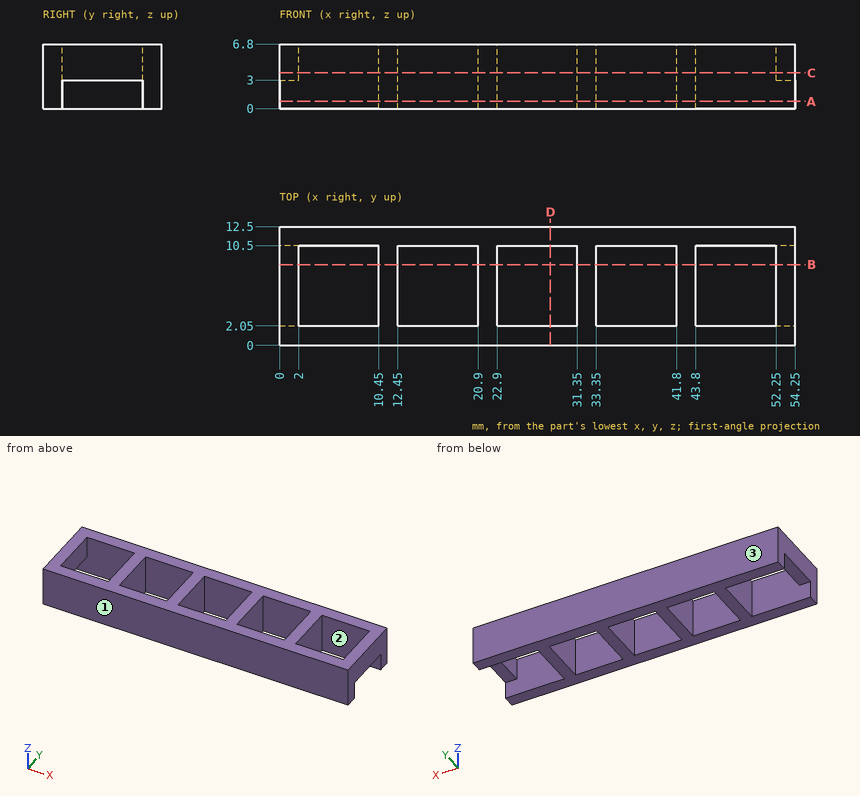
Verification items for this drawing (mm, ordinates from the low corner). Give positions to 0.01 mm unless a question says otherwise; leave off trailing zeros. Write each loop counter-clockwise with the first axis right and the second up, starting at its lowest first coordinate (ties: lowest second). Pieces come first, ordered by that corner, then holes.
1) Release check for a two-part mould opening along Y. For the marked faces 1, 2 and 3 record: pulls with the +Y half, pulls with the -Y half, needs draft (parallel to the pull), parting line crosses it, or undercut.
2) Section check A-A, the plane z = 0.75. Record the boundary of the cut face in (x, y).
3) Section check D-D, the plane x = 28.5. Record the boundary of the cut face in (y, z).
4) Section check B-B, the plane y = 8.5. Record the boundary of the cut face in (x, z).
5) Section check C-C, the plane z = 3.75. Record the boundary of the cut face in (x, y).
6) Gauge pin test, flat ends, axial feed: pin 1 (1 mm diameter, centred on y = 9, z = 3.5, fed in from -X); pin 2 (5 mm diameter, centred on x = 6.5, y = 6.5, fed in from +Z); pin 3 (1 mm diameter, centred on x = 1, y = 7, fed in from -Z). Record the tip position at first contact, or that the pin passes through.
7) Material ranges on L1, parallel to X at y = 5.25, z = 0.75; L2, parallel to X at y = 8, z = 3.5; L3, parallel to Y at x = 14, z = 4, recorded low to high.
Computed:
1. face 1: pulls with the -Y half
1. face 2: undercut
1. face 3: pulls with the +Y half
2. outline: (0, 0) - (54.25, 0) - (54.25, 2.05) - (43.8, 2.05) - (43.8, 10.5) - (54.25, 10.5) - (54.25, 12.5) - (0, 12.5) - (0, 10.5) - (10.45, 10.5) - (10.45, 2.05) - (0, 2.05) - close; hole (12.45, 2.05) - (20.9, 2.05) - (20.9, 10.5) - (12.45, 10.5) - close; hole (22.9, 2.05) - (31.35, 2.05) - (31.35, 10.5) - (22.9, 10.5) - close; hole (33.35, 2.05) - (41.8, 2.05) - (41.8, 10.5) - (33.35, 10.5) - close
3. outline: (0, 0) - (2.05, 0) - (2.05, 6.8) - (0, 6.8) - close; (10.5, 0) - (12.5, 0) - (12.5, 6.8) - (10.5, 6.8) - close
4. outline: (0, 3) - (2, 3) - (2, 6.8) - (0, 6.8) - close; (10.45, 0) - (12.45, 0) - (12.45, 6.8) - (10.45, 6.8) - close; (20.9, 0) - (22.9, 0) - (22.9, 6.8) - (20.9, 6.8) - close; (31.35, 0) - (33.35, 0) - (33.35, 6.8) - (31.35, 6.8) - close; (41.8, 0) - (43.8, 0) - (43.8, 6.8) - (41.8, 6.8) - close; (52.25, 3) - (54.25, 3) - (54.25, 6.8) - (52.25, 6.8) - close
5. outline: (0, 0) - (54.25, 0) - (54.25, 12.5) - (0, 12.5) - close; hole (2, 2.05) - (10.45, 2.05) - (10.45, 10.5) - (2, 10.5) - close; hole (12.45, 2.05) - (20.9, 2.05) - (20.9, 10.5) - (12.45, 10.5) - close; hole (22.9, 2.05) - (31.35, 2.05) - (31.35, 10.5) - (22.9, 10.5) - close; hole (33.35, 2.05) - (41.8, 2.05) - (41.8, 10.5) - (33.35, 10.5) - close; hole (43.8, 2.05) - (52.25, 2.05) - (52.25, 10.5) - (43.8, 10.5) - close
6. pin 1: stops at x = 0
6. pin 2: passes through
6. pin 3: stops at z = 3
7. L1: x = 10.45 to 12.45, 20.9 to 22.9, 31.35 to 33.35, 41.8 to 43.8
7. L2: x = 0 to 2, 10.45 to 12.45, 20.9 to 22.9, 31.35 to 33.35, 41.8 to 43.8, 52.25 to 54.25
7. L3: y = 0 to 2.05, 10.5 to 12.5
